from build123d import *

# Parameters (mm, degrees)
SKETCH1_W           = 30
SKETCH1_H           = 30
BOSS_EXTRUDE1_DEPTH = 20
SKETCH1_6_W         = 14
SKETCH1_6_H         = 14
CUT_EXTRUDE1_DEPTH  = 15
SKETCH1_7_W         = 10
SKETCH1_7_H         = 10
SKETCH1_7_H_2       = 3
SKETCH1_7_W_2       = 3
BOSS_EXTRUDE2_DEPTH = 15


with BuildPart() as part:
    # Sketch1 → Boss-Extrude1 (new body)
    with BuildSketch(Plane(origin=(0, 0, 0), x_dir=(1, 0, 0), z_dir=(0, 1, 0))):
        Rectangle(SKETCH1_W, SKETCH1_H)
    extrude(amount=-BOSS_EXTRUDE1_DEPTH)

    # Sketch1_6 → Cut-Extrude1 (cut)
    with BuildSketch(Plane(origin=(0, 0, 0), x_dir=(1, 0, 0), z_dir=(0, 1, 0))):
        Polygon((2, 1), (12, 1), (12, 12), (12, 15), (2, 15), align=None)
        Polygon((-12, -12), (-1, -12), (-1, -2), (-15, -2), (-15, -12), align=None)
        with Locations((-8, 8)):
            Rectangle(SKETCH1_6_W, SKETCH1_6_H)
    extrude(amount=-CUT_EXTRUDE1_DEPTH, mode=Mode.SUBTRACT)

    # Sketch1_7 → Boss-Extrude2 (add)
    with BuildSketch(Plane(origin=(0, 0, 0), x_dir=(1, 0, 0), z_dir=(0, 1, 0))):
        with Locations((7, -7)):
            Rectangle(SKETCH1_7_W, SKETCH1_7_H)
        with Locations((7, -0.5)):
            Rectangle(SKETCH1_7_W, SKETCH1_7_H_2)
        with Locations((0.5, -7)):
            Rectangle(SKETCH1_7_W_2, SKETCH1_7_H)
        with Locations((0.5, -0.5)):
            Rectangle(SKETCH1_7_W_2, SKETCH1_7_H_2)
    extrude(amount=BOSS_EXTRUDE2_DEPTH)


solid = part.part
Verification items for the finished model (mm, model axes). A direction names the side the tool comes from. Round coordinates to 2 decimals unless told otherwise and drop trailing zeros. Loops run counter-clockwise (first coordinate to the right, second up) from the corner with the lowest first, then second, coordinate; pieces in that order, holes last. Notation, with made-up numbers: M 30.5,38.25 L 71.5,38.25 A27 cw 71.5,71.25 Z; hole C -19.75,-3 d3. An arc over 180 degrees is marked long. Write each question's results on one line, items separated by ' | '.
1) Section check B-B on x = 2.5. Record the boundary of the cut face in (y, z), then the cut area to 3 significant figures.
Checks:
outline: M -20,-15 L -15,-15 L -15,-1 L 15,-1 L 15,12 L 0,12 L 0,15 L -20,15 Z | area: 585 mm2
2) Mould release check, pull along Z, two halves, no side actions. Record for faces 5 (the flat face through (0, 0, -8)), 6 (the flat face through (0, -14, -15)), 7 (the flat face through (-8, -7, 2)): released by +Z, released by -Z, zero draft, split by the parting line, or undercut.
Checks:
face 5: zero draft | face 6: released by -Z | face 7: undercut
3) Scan lines: L1, parallel to X at y = -10, z = -8.25; L2, parallel to Z at x = 3.25, y = -13. Record each from-to range of solid material in increasing order. Write a range as from..to.
Checks:
L1: x = -1..2, 12..15 | L2: z = -1..15
4) Section check D-D on x = -4.5. Record the boundary of the cut face in (y, z).
Checks:
outline: M -20,-15 L -15,-15 L -15,-1 L 0,-1 L 0,2 L -15,2 L -15,12 L 0,12 L 0,15 L -20,15 Z
5) Access from +Z, -Z, +X, -X, +Y, -Y to the whole of each face (thin tool, end or side, straight path). Record for faces 1 (the flat face through (-1, -7, -8)), 2 (the flat face through (2, -7, -8)), 3 (the flat face through (12, 7, 6)), 4 (the flat face through (-8, 0, 0)).
Checks:
face 1: -Z, -X, +Y | face 2: -Z, +Y | face 3: +Z, -Z, +X, +Y | face 4: +Z, -Z, -X, +Y
6) Gauge pin test, flat ends, axial feed: P1, Ø6, axis at x = -11, z = 2, coming from the +Y side; P2, Ø8, axis at y = 2.5, z = 1.5, coming from the -X side; P3, Ø6.5, axis at y = 6.5, z = 6, coming from the -X side; P4, Ø4, axis at x = 6, y = -1.5, coming from the -Z side. Record the tip position at first contact, or that the pin passes through.
Checks:
P1: stops at y = 0 | P2: stops at x = -15 | P3: stops at x = -1 | P4: stops at z = -1
7) Section check C-C on z = 3.25. Record the boundary of the cut face in (x, y), then the cut area to 3 significant figures.
Checks:
outline: M -15,-20 L 15,-20 L 15,0 L 12,0 L 12,15 L -1,15 L -1,-15 L -15,-15 Z | area: 585 mm2
8) Section check A-A on y = -7.5. Record the boundary of the cut face in (x, z), then the cut area to 3 significant figures.
Checks:
outline: M -15,-1 L -1,-1 L -1,-15 L 2,-15 L 2,-1 L 12,-1 L 12,-15 L 15,-15 L 15,15 L -15,15 L -15,12 L -1,12 L -1,2 L -15,2 Z | area: 424 mm2
